from build123d import *

# Parameters (mm, degrees)
F1_DEPTH = 60
F3_DEPTH = 20.001
F5_DEPTH = 20.001
F7_DEPTH = 20.001


with BuildPart() as f1:
    # F0 (on Front) → F1 (new body)
    with BuildSketch(Plane.XZ):
        Polygon((0, 60), (0, 0), (90, 0), (90, 20), (20, 20), (20, 60), align=None)
    extrude(amount=F1_DEPTH)

    # F2 (on face) → F3 (cut, through all)
    with BuildSketch(Plane.YZ.offset(20)):
        with BuildLine():
            Line((-20, 60), (-40, 60))
            Line((-40, 60), (-40, 40))
            ThreePointArc((-40, 40), (-30, 30), (-20, 40))
            Line((-20, 40), (-20, 60))
        make_face()
    extrude(amount=-F3_DEPTH, mode=Mode.SUBTRACT)

    # F4 (on face) → F5 (cut, through all)
    with BuildSketch(Plane.XY.offset(20)):
        Polygon((90, -60), (90, -30), (40, -60), align=None)
    extrude(amount=-F5_DEPTH, mode=Mode.SUBTRACT)

    # F6 (on face) → F7 (cut, through all)
    with BuildSketch(Plane.XY.offset(20)):
        with BuildLine():
            ThreePointArc((40, -10), (30, -20), (40, -30))
            Line((40, -30), (60, -30))
            ThreePointArc((60, -30), (70, -20), (60, -10))
            Line((60, -10), (40, -10))
        make_face()
    extrude(amount=-F7_DEPTH, mode=Mode.SUBTRACT)


solid = f1.part
The model under review builds one solid part; all positions refer to its coordinate system, in mm. A direction names the side the tool comes from. Give positions to 0.01 mm unless a question says otherwise; leave off trailing zeros. Write each loop counter-clockwise with the first axis right and the second up, starting at its lowest first coordinate (ties: lowest second). Pieces come first, ordered by that corner, then holes. Notation, with made-up numbers: M -24.5,-36 L 30.5,-36 A20 ccw 30.5,-8 Z; hole C -27.5,49 d10. An arc over 180 degrees is marked long. One line per question, with ' | ' between items. Start each with the question number.
Item 1: We need section B-B on y = -14. Write out the cut boundary in (x, z).
Item 2: We need section D-D on x = 32. Write out the cut boundary in (y, z).
Item 3: Wall thickness on line 1 (Y direction, x = 6.5, z = 49); line 2 (X direction, y = -51.5, z = 41): over which ranges is each line inside the solid? List them lowest first. Write a range as from..to.
Item 4: We need section C-C on z = 9. Write out the cut boundary in (x, y).
Item 5: For faces 5 (the flat face through (50, -30, 10)), 6 (the flat face through (10, -40, 50)), 7 (the flat face through (55, -36, 20)), list the 3-axis set-ups (+Z, -Z, +X, -X, +Y, -Y) from which the entire face can be reached by the end or side of a thin tool; tool diameter is ignored.
Item 6: We need section A-A on x = 54.5. Write out the cut boundary in (y, z).
Item 7: For pin 1 (12 mm diameter, centred on x = 47.5, y = -51, fed in from +Z); pin 2 (16 mm diameter, centred on x = 49, z = 12.5, fed in from -Y), all flat-tipped, find the tip position at first contact; note any pin that passes through.
Item 8: Draft analysis for pull direction X (two halves, no side actions). For faces 1 (the flat face through (50, -10, 10)), 2 (the flat face through (10, -50, 60)), 3 (the cylindrical face through (70, -20, 10)), 4 (the flat face through (0, -30, 24)), state which applies: released by +X, released by -X, zero draft, split by the parting line, or undercut.
Results found:
1) outline: M 0,0 L 32,0 L 32,20 L 20,20 L 20,60 L 0,60 Z; M 68,0 L 90,0 L 90,20 L 68,20 Z
2) outline: M -60,0 L -26,0 L -26,20 L -60,20 Z; M -14,0 L 0,0 L 0,20 L -14,20 Z
3) line 1: y = -60..-40, -20..0 | line 2: x = 0..20
4) outline: M 0,-60 L 40,-60 L 90,-30 L 90,0 L 0,0 Z; hole M 40,-30 L 60,-30 A10 ccw 60,-10 L 40,-10 A10 ccw Z
5) face 5: +Z, -Z | face 6: +Z, +X, -X | face 7: +Z, +X, +Y, -Y
6) outline: M -51.3,0 L -30,0 L -30,20 L -51.3,20 Z; M -10,0 L 0,0 L 0,20 L -10,20 Z
7) pin 1: stops at z = 20 | pin 2: stops at y = -59.4
8) face 1: undercut | face 2: zero draft | face 3: undercut | face 4: released by -X
